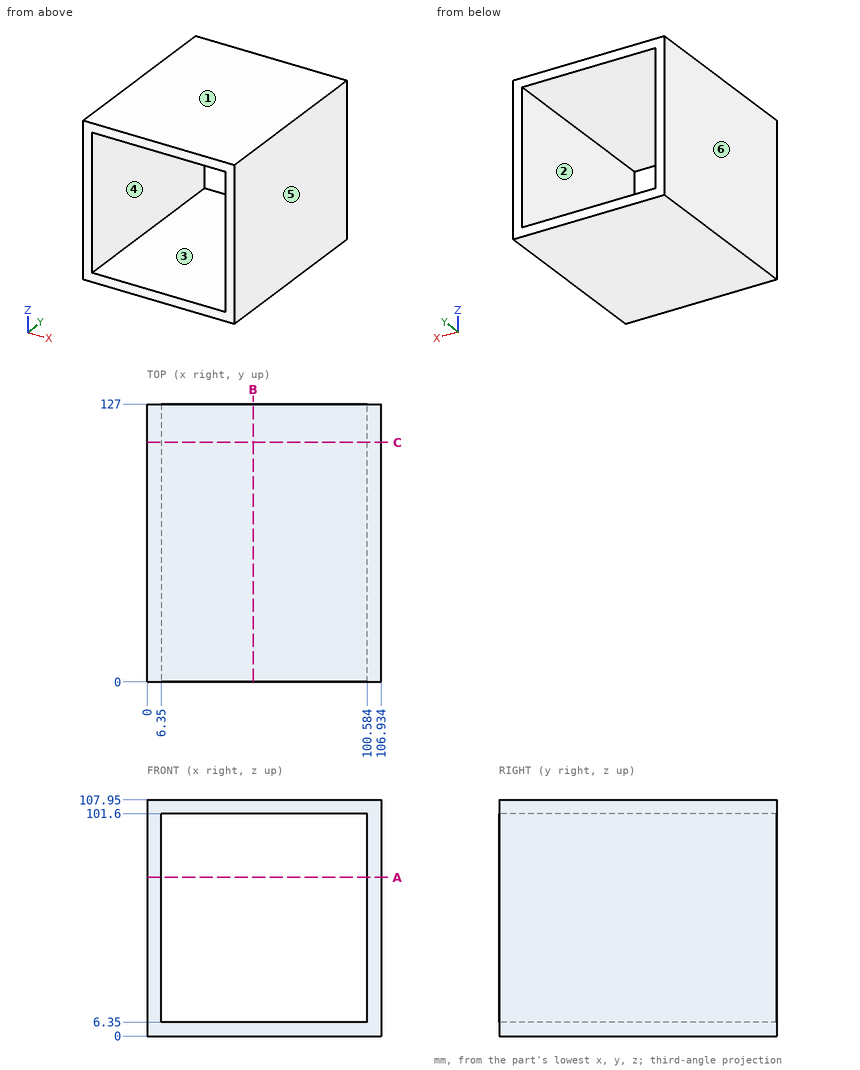
Study the drawing (mm; zero at the part's minimum x, y, z) and answer. A direction names the side the tool comes from. Round coordinates to 2 decimals unless told otherwise and drop trailing zeros. Write each loop counter-clockwise with the first axis right and the second up, starting at its lowest first coordinate (ties: lowest second). Pieces come first, ordered by that corner, then holes. Notation, with made-up numbers: (24.5, 29.5) - (67.5, 29.5) arc R9 cw to (67.5, 36.5) - close; hole circle Ø10 at (86.5, 46). An arc over 180 degrees is marked (long way). Use a Markdown table: item, result. Add a question column.
1. The part is cut by section B-B (x = 48.5). Write down the section's boundary in (y, z), and give its area (3 significant figures).
2. For a pull along X with two mould halves and no side action, classify the marked faces 3, 4, 5 and 6 as +X half, -X half, draft (parallel to the pull), parting line (faces both ways), or undercut.
3. Consider line 1 (Z direction, x = 20.5, y = 11.5); line 2 (X direction, y = 27.5, z = 19.5). Determine where each line is inside the solid, lowest interval first.
4. The part is cut by section A-A (z = 72.5). Write down the section's boundary in (x, y), and give its area (3 significant figures).
5. Flat-ended cylindrical pins translate along their axes: P1, Ø12, axis at x = 16.5, z = 51, coming from the -Y side; P2, Ø3, axis at x = 93.5, y = 101.5, coming from the -Z side. Find the tip coordinate at first contact, or state that the pin passes through.
6. A tool of negligible diameter and unlimited length cuts with its end or side. For the marked faces 1 and 2, from which of +Z, -Z, +X, -X, +Y, -Y can it reach the whole face along a straight path? Write none if from no direction.
7. The part is cut by section C-C (y = 109.5). Write down the section's boundary in (x, z).
Reported:
| question | item | result |
|---|---|---|
| 1 | outline | (0, 0) - (127, 0) - (127, 6.35) - (0, 6.35) - close; (0, 101.6) - (127, 101.6) - (127, 107.95) - (0, 107.95) - close |
| 1 | area | 1,610 mm^2 |
| 2 | face 3 | undercut |
| 2 | face 4 | undercut |
| 2 | face 5 | +X half |
| 2 | face 6 | -X half |
| 3 | line 1 | 0 to 6.35, 101.6 to 107.95 |
| 3 | line 2 | 0 to 6.35, 100.58 to 106.93 |
| 4 | outline | (0, 0) - (6.35, 0) - (6.35, 127) - (0, 127) - close; (100.58, 0) - (106.93, 0) - (106.93, 127) - (100.58, 127) - close |
| 4 | area | 1,610 mm^2 |
| 5 | P1 | through |
| 5 | P2 | z = 0 |
| 6 | face 1 | +Z, +X, -X, +Y, -Y |
| 6 | face 2 | +Y, -Y |
| 7 | outline | (0, 0) - (106.93, 0) - (106.93, 107.95) - (0, 107.95) - close; hole (6.35, 6.35) - (100.58, 6.35) - (100.58, 101.6) - (6.35, 101.6) - close |
